from build123d import *

# Parameters (mm, degrees)
MODEL_R             = 1.632
MODEL_R_2           = 3.5
BOSS_EXTRUDE1_DEPTH = 6.35


with BuildPart() as part:
    # Model → Boss-Extrude1 (new body)
    with BuildSketch(Plane.XY):
        with BuildLine():
            ThreePointArc((-16.948506407, 1.322168893), (-14.884445144, 0.075680968), (-12.496345641, -0.2575784))
            ThreePointArc((-12.496345641, -0.2575784), (-12.43052917, -1.306501262), (-12.276824067, -2.346186657))
            ThreePointArc((-12.276824067, -2.346186657), (-14.543449347, -3.168677314), (-16.303246508, -4.817068954))
            ThreePointArc((-16.303246508, -4.817068954), (-16.167960777, -5.253288904), (-16.021005579, -5.685717215))
            ThreePointArc((-16.021005579, -5.685717215), (-13.628399474, -5.984911247), (-11.311213223, -5.318031254))
            ThreePointArc((-11.311213223, -5.318031254), (-10.824451522, -6.2495), (-10.261156776, -7.136782372))
            ThreePointArc((-10.261156776, -7.136782372), (-11.997284916, -8.810084533), (-12.934478336, -11.031739218))
            ThreePointArc((-12.934478336, -11.031739218), (-12.633462033, -11.375220308), (-12.32332734, -11.710491163))
            ThreePointArc((-12.32332734, -11.710491163), (-10.015879724, -11.010657936), (-8.170269281, -9.458948191))
            ThreePointArc((-8.170269281, -9.458948191), (-7.346727868, -10.111903413), (-6.471242258, -10.693363579))
            ThreePointArc((-6.471242258, -10.693363579), (-7.376680931, -12.9281481), (-7.329221354, -15.338921551))
            ThreePointArc((-7.329221354, -15.338921551), (-6.914522932, -15.53027278), (-6.49483385, -15.710414802))
            ThreePointArc((-6.49483385, -15.710414802), (-4.671523379, -14.13256184), (-3.616611555, -11.964327054))
            ThreePointArc((-3.616611555, -11.964327054), (-2.598688224, -12.225866862), (-1.562391165, -12.400965077))
            ThreePointArc((-1.562391165, -12.400965077), (-1.480581798, -14.810817411), (-0.456675416, -16.993864998))
            ThreePointArc((-0.456675416, -16.993864998), (0, -17), (0.456675416, -16.993864998))
            ThreePointArc((0.456675416, -16.993864998), (1.480581798, -14.810817411), (1.562391165, -12.400965077))
            ThreePointArc((1.562391165, -12.400965077), (2.598688224, -12.225866862), (3.616611555, -11.964327054))
            ThreePointArc((3.616611555, -11.964327054), (4.671523379, -14.13256184), (6.49483385, -15.710414802))
            ThreePointArc((6.49483385, -15.710414802), (6.914522932, -15.53027278), (7.329221354, -15.338921551))
            ThreePointArc((7.329221354, -15.338921551), (7.376680931, -12.9281481), (6.471242258, -10.693363579))
            ThreePointArc((6.471242258, -10.693363579), (7.346727868, -10.111903413), (8.170269281, -9.458948191))
            ThreePointArc((8.170269281, -9.458948191), (10.015879724, -11.010657936), (12.32332734, -11.710491163))
            ThreePointArc((12.32332734, -11.710491163), (12.633462033, -11.375220308), (12.934478336, -11.031739218))
            ThreePointArc((12.934478336, -11.031739218), (11.997284916, -8.810084533), (10.261156776, -7.136782372))
            ThreePointArc((10.261156776, -7.136782372), (10.824451522, -6.2495), (11.311213223, -5.318031254))
            ThreePointArc((11.311213223, -5.318031254), (13.628399474, -5.984911247), (16.021005579, -5.685717215))
            ThreePointArc((16.021005579, -5.685717215), (16.167960777, -5.253288904), (16.303246508, -4.817068954))
            ThreePointArc((16.303246508, -4.817068954), (14.543449347, -3.168677314), (12.276824067, -2.346186657))
            ThreePointArc((12.276824067, -2.346186657), (12.43052917, -1.306501262), (12.496345641, -0.2575784))
            ThreePointArc((12.496345641, -0.2575784), (14.884445144, 0.075680968), (16.948506407, 1.322168893))
            ThreePointArc((16.948506407, 1.322168893), (16.906872221, 1.776983876), (16.853035248, 2.230516294))
            ThreePointArc((16.853035248, 2.230516294), (14.574919264, 3.020622999), (12.169716946, 2.850086045))
            ThreePointArc((12.169716946, 2.850086045), (11.887255397, 3.862403413), (11.520746371, 4.847412099))
            ThreePointArc((11.520746371, 4.847412099), (13.566835028, 6.123187257), (14.945456505, 8.101439987))
            ThreePointArc((14.945456505, 8.101439987), (14.722431864, 8.5), (14.488781088, 8.892425011))
            ThreePointArc((14.488781088, 8.892425011), (12.08625323, 8.687630155), (9.958355206, 7.553552978))
            ThreePointArc((9.958355206, 7.553552978), (9.288567174, 8.363463449), (8.553105391, 9.114241009))
            ThreePointArc((8.553105391, 9.114241009), (9.903395884, 11.111938841), (10.358201398, 13.479898509))
            ThreePointArc((10.358201398, 13.479898509), (9.992349289, 13.753288904), (9.619285053, 14.016752658))
            ThreePointArc((9.619285053, 14.016752658), (7.507764213, 12.852467132), (6.025103383, 10.950941979))
            ThreePointArc((6.025103383, 10.950941979), (5.083801302, 11.418404675), (4.106554786, 11.805134848))
            ThreePointArc((4.106554786, 11.805134848), (4.527569623, 14.179335251), (3.979919168, 16.527560117))
            ThreePointArc((3.979919168, 16.527560117), (3.534498744, 16.628509212), (3.086527243, 16.717456433))
            ThreePointArc((3.086527243, 16.717456433), (1.631114557, 14.794995781), (1.050056448, 12.454813626))
            ThreePointArc((1.050056448, 12.454813626), (0, 12.499), (-1.050056448, 12.454813626))
            ThreePointArc((-1.050056448, 12.454813626), (-1.631114557, 14.79499578), (-3.086527243, 16.717456433))
            ThreePointArc((-3.086527243, 16.717456433), (-3.534498744, 16.628509212), (-3.979919168, 16.527560117))
            ThreePointArc((-3.979919168, 16.527560117), (-4.527569623, 14.179335251), (-4.106554786, 11.805134848))
            ThreePointArc((-4.106554786, 11.805134848), (-5.083801302, 11.418404675), (-6.025103383, 10.950941979))
            ThreePointArc((-6.025103383, 10.950941979), (-7.507764213, 12.852467132), (-9.619285053, 14.016752658))
            ThreePointArc((-9.619285053, 14.016752658), (-9.992349289, 13.753288904), (-10.358201398, 13.479898509))
            ThreePointArc((-10.358201398, 13.479898509), (-9.903395884, 11.111938841), (-8.553105391, 9.114241009))
            ThreePointArc((-8.553105391, 9.114241009), (-9.288567174, 8.363463449), (-9.958355206, 7.553552978))
            ThreePointArc((-9.958355206, 7.553552978), (-12.08625323, 8.687630155), (-14.488781088, 8.892425011))
            ThreePointArc((-14.488781088, 8.892425011), (-14.722431864, 8.5), (-14.945456505, 8.101439987))
            ThreePointArc((-14.945456505, 8.101439987), (-13.566835028, 6.123187257), (-11.520746371, 4.847412099))
            ThreePointArc((-11.520746371, 4.847412099), (-11.887255397, 3.862403413), (-12.169716946, 2.850086045))
            ThreePointArc((-12.169716946, 2.850086045), (-14.574919264, 3.020622999), (-16.853035248, 2.230516294))
            ThreePointArc((-16.853035248, 2.230516294), (-16.906872221, 1.776983876), (-16.948506407, 1.322168893))
        make_face()
        with Locations((-4.7625, -8.248891971)):
            Circle(MODEL_R, mode=Mode.SUBTRACT)
        with Locations((4.7625, -8.248891971)):
            Circle(MODEL_R, mode=Mode.SUBTRACT)
        with Locations((9.525, 0)):
            Circle(MODEL_R, mode=Mode.SUBTRACT)
        with Locations((4.7625, 8.248891971)):
            Circle(MODEL_R, mode=Mode.SUBTRACT)
        with Locations((-4.7625, 8.248891971)):
            Circle(MODEL_R, mode=Mode.SUBTRACT)
        with Locations((-9.525, 0)):
            Circle(MODEL_R, mode=Mode.SUBTRACT)
        Circle(MODEL_R_2, mode=Mode.SUBTRACT)
    extrude(amount=BOSS_EXTRUDE1_DEPTH)


solid = part.part
Source: CAD feature listing. Evaluate the final solid. Frame: model axes, mm. A direction names the side the tool comes from. Coordinates: 2 decimals unless noted, no trailing zeros. Order: outer loops, then holes, each group sorted by start corner. A loop starts at its lowest first (then second) coordinate and runs counter-clockwise, first axis right, second up. Notation, with made-up numbers: M 42.5,24 L 97.5,24 A32 cw 97.5,54 Z; hole C 64,29 d11. An arc over 180 degrees is marked long. Write each question's results on one line, items separated by ' | '. Start each with the question number.
1. Pin query (flat end, axial travel): pin 1 (3 mm diameter, centred on x = -2.5, z = 5.5, fed in from -Y); pin 2 (1.5 mm diameter, centred on y = 0, z = 3.5, fed in from +X). Return the tip coordinate at first contact, or that it passes through.
2. Section A-A, the plane x = 0. Return the cut outline in (y, z).
3. Section C-C, the plane x = -5. Return the cut outline in (y, z).
4. Reachability of faces 1 (the face through (4.651, -14.106, 3.131)), 2 (the face through (7.53, 12.87, 3.13)), 3 (the face through (4.53, 14.15, 3.13)) from +Z, -Z, +X, -X, +Y, -Y: full face, straight path, thin tool, end or side. Return the list, or none.
5. Section B-B, the plane y = -3. Return the cut outline in (x, z), then the cut area to 3 significant figures.
6. Section D-D, the plane y = 0.5. Return the cut outline in (x, z).
7. Draft query along Y for faces 4 (the face through (-9.28, 8.37, 3.13)), 5 (the face through (0, -17, 3)), 6 (the face through (-3.53, 16.63, 3.13)), 7 (the face through (-7.37, -12.89, 3.13)). Return one class per face: +Y half, -Y half, draft (parallel to the pull), parting line (faces both ways), or undercut.
8. Material intervals for L1, parallel to X at y = 1, z = 4.25; L2, parallel to X at y = -10, z = 5.5; L3, parallel to Y at x = -13, z = 0.5, sorted ascending.
Solution:
1) pin 1: y = -16.12 | pin 2: x = 16.22
2) outline: M -17,0 L -3.5,0 L -3.5,6.35 L -17,6.35 Z; M 3.5,0 L 12.5,0 L 12.5,6.35 L 3.5,6.35 Z
3) outline: M -14.52,0 L -9.86,0 L -9.86,6.35 L -14.52,6.35 Z; M -6.63,0 L 6.63,0 L 6.63,6.35 L -6.63,6.35 Z; M 9.86,0 L 11.46,0 L 11.46,6.35 L 9.86,6.35 Z
4) face 1: +Z, -Z, -Y | face 2: +Z, -Z, +Y | face 3: +Z, -Z
5) outline: M -14.25,0 L -1.8,0 L -1.8,6.35 L -14.25,6.35 Z; M 1.8,0 L 14.25,0 L 14.25,6.35 L 1.8,6.35 Z | area: 158 mm²
6) outline: M -15.82,0 L -11.08,0 L -11.08,6.35 L -15.82,6.35 Z; M -7.97,0 L -3.46,0 L -3.46,6.35 L -7.97,6.35 Z; M 3.46,0 L 7.97,0 L 7.97,6.35 L 3.46,6.35 Z; M 11.08,0 L 15.82,0 L 15.82,6.35 L 11.08,6.35 Z
7) face 4: undercut | face 5: -Y half | face 6: +Y half | face 7: undercut
8) L1: -16.57 to -10.81, -8.24 to -3.35, 3.35 to 8.24, 10.81 to 16.57 | L2: -12.63 to -8.65, -7.5 to 7.5, 8.65 to 12.63 | L3: -5.9 to -2.5, -0.27 to 3.02, 5.65 to 8.88
